from build123d import *

# Parameters (mm, degrees)
SKETCH1_W           = 50
SKETCH1_H           = 50
BOSS_EXTRUDE1_DEPTH = 30
BOSS_EXTRUDE2_DEPTH = 20
BOSS_EXTRUDE3_DEPTH = 20
CUT_EXTRUDE5_DEPTH  = 20
CUT_EXTRUDE6_DEPTH  = 20
CHAMFER1_SIZE       = 2
SKETCH4_R           = 3.1
CUT_EXTRUDE4_DEPTH  = 4
CHAMFER2_SIZE       = 1
CHAMFER3_SIZE       = 0.75
CHAMFER4_SIZE       = 2.5


with BuildPart() as part:
    # Sketch1 → Boss-Extrude1 (new body)
    with BuildSketch(Plane(origin=(0, 0, 0), x_dir=(1, 0, 0), z_dir=(0, 1, 0))):
        with Locations((25, 25)):
            Rectangle(SKETCH1_W, SKETCH1_H)
    extrude(amount=BOSS_EXTRUDE1_DEPTH)

    # Sketch3 → Boss-Extrude2 (add)
    with BuildSketch(Plane(origin=(0, 0, 0), x_dir=(1, 0, 0), z_dir=(0, 1, 0))):
        Polygon((50, 16.674315781), (50, 33.325684219), (52.3, 34.653589838), (52.3, 15.346410162), align=None)
    extrude(amount=BOSS_EXTRUDE2_DEPTH)

    # Sketch3_3 → Boss-Extrude3 (add)
    with BuildSketch(Plane(origin=(0, 0, 0), x_dir=(1, 0, 0), z_dir=(0, 1, 0))):
        Polygon((33.325684219, 50), (16.674315781, 50), (15.346410162, 52.3), (34.653589838, 52.3), align=None)
    extrude(amount=BOSS_EXTRUDE3_DEPTH)

    # Sketch3_6 → Cut-Extrude5 (cut)
    with BuildSketch(Plane(origin=(0, 0, 0), x_dir=(1, 0, 0), z_dir=(0, 1, 0))):
        Polygon((0, 33.787564435), (2.7, 35.346410162), (2.7, 14.653589838), (0, 16.212435565), align=None)
    extrude(amount=CUT_EXTRUDE5_DEPTH, mode=Mode.SUBTRACT)

    # Sketch3_7 → Cut-Extrude6 (cut)
    with BuildSketch(Plane(origin=(0, 0, 0), x_dir=(1, 0, 0), z_dir=(0, 1, 0))):
        Polygon((16.212435565, 0), (14.653589838, 2.7), (35.346410162, 2.7), (33.787564435, 0), align=None)
    extrude(amount=CUT_EXTRUDE6_DEPTH, mode=Mode.SUBTRACT)

    # Chamfer1
    chamfer1_edges = [part.edges().sort_by_distance(p)[0] for p in [
        (50, 30, -25),
        (25, 30, -50),
        (0, 30, -25),
        (25, 30, 0),
    ]]
    chamfer(chamfer1_edges, length=CHAMFER1_SIZE)

    # Sketch4 → Cut-Extrude4 (cut)
    with BuildSketch(Plane(origin=(0, 0, 0), x_dir=(1, 0, 0), z_dir=(0, 1, 0))):
        with Locations(Location((12.5, 37.5, 0), (0, 0, 270))):
            Circle(SKETCH4_R)
        with Locations(Location((37.5, 37.5, 0), (0, 0, 270))):
            Circle(SKETCH4_R)
        with Locations(Location((37.5, 12.5, 0), (0, 0, 270))):
            Circle(SKETCH4_R)
        with Locations(Location((12.5, 12.5, 0), (0, 0, 270))):
            Circle(SKETCH4_R)
    extrude(amount=CUT_EXTRUDE4_DEPTH, mode=Mode.SUBTRACT)

    # Chamfer2
    chamfer2_edges = [part.edges().sort_by_distance(p)[0] for p in [
        (12.5, 4, -15.6),
        (37.5, 4, -15.6),
        (37.5, 4, -40.6),
        (12.5, 4, -40.6),
    ]]
    chamfer(chamfer2_edges, length=CHAMFER2_SIZE)

    # Chamfer3
    chamfer3_edges = [part.edges().sort_by_distance(p)[0] for p in [
        (50, 0, -41.66284211),
        (51.15, 0, -16.010362971),
        (51.15, 0, -33.989637029),
        (52.3, 0, -25),
        (8.33715789, 0, -50),
        (33.989637029, 0, -51.15),
        (16.010362971, 0, -51.15),
        (25, 0, -52.3),
        (0, 0, -8.106217783),
        (1.35, 0, -15.433012702),
        (1.35, 0, -34.566987298),
        (2.7, 0, -25),
        (41.66284211, 0, -50),
        (41.893782217, 0, 0),
        (50, 0, -8.33715789),
        (34.566987298, 0, -1.35),
        (15.433012702, 0, -1.35),
        (8.106217783, 0, 0),
        (25, 0, -2.7),
        (0, 0, -41.893782217),
        (12.5, 0, -15.6),
        (37.5, 0, -15.6),
        (37.5, 0, -40.6),
        (12.5, 0, -40.6),
    ]]
    chamfer(chamfer3_edges, length=CHAMFER3_SIZE)

    # Chamfer4
    chamfer4_edges = [part.edges().sort_by_distance(p)[0] for p in [
        (0, 20, -25),
        (25, 20, 0),
    ]]
    chamfer(chamfer4_edges, length=CHAMFER4_SIZE)


solid = part.part
Model file for the job. Use its own axes, mm. A direction names the side the tool comes from. Coordinates: 2 decimals unless noted, no trailing zeros. Order: outer loops, then holes, each group sorted by start corner. A loop starts at its lowest first (then second) coordinate and runs counter-clockwise, first axis right, second up. Notation, with made-up numbers: (73, 11.5) -> (100, 11.5) arc R25 ccw to (100, 44.5) -> close; hole circle Ø2 at (12, 86.25). An arc over 180 degrees is marked (long way). Return JSON: item names as keys, results as strings. Group by question number.
Item 1: Saw through at D-D on x = 6.5. Write the cut outline in (y, z), then the cut area to 3 significant figures.
Item 2: Saw through at C-C on y = 7. Write the cut outline in (x, z).
Item 3: Saw through at B-B on x = 24. Write the cut outline in (y, z), then the cut area to 3 significant figures.
Item 4: Pull direction Z, two halves, no side cores. Call faces 1 (the flat face through (50.75, 0.38, -33.33)), 2 (the flat face through (1.331, 11.473, -34.556)), 3 (the flat face through (25, 20, -51)): pulls with the +Z half, pulls with the -Z half, needs draft (parallel to the pull), parting line crosses it, or undercut.
Item 5: Wall check: line 1 along X through (y, z) = (1.9, -12.5); line 2 along Z through (x, y) = (16, 5.5); line 3 along X through (y, z) = (13, -38.5). Give the ranges that are in metal, low to high. Write a range as [from, to].
Item 6: Tool access for faces 4 (the cylindrical face through (13.431, 1.859, -34.543)), 5 (the flat face through (25, 29, -1)): list every direction of +Z, -Z, +X, -X, +Y, -Y with a clear straight run to the whole face (end or side of a thin tool).
Item 7: Flat gauge pins, fed straight in: P1, Ø5, axis at x = 37.5, z = -37.5, coming from the -Y side; P2, Ø1.3, axis at x = 11.5, z = -38.5, coming from the -Y side; P3, Ø2.5, axis at x = 50.5, z = -27, coming from the +Y side. Where does each tip first touch, or does it go through?
Item 8: Saw through at A-A on z = -37.5. Write the cut outline in (x, y).
Values found:
{
 "1": {"outline": "(0, -49.25) -> (0.75, -50) -> (28, -50) -> (30, -48) -> (30, -2) -> (28, 0) -> (0.75, 0) -> (0, -0.75) -> close", "area": "1,500 mm2"},
 "2": {"outline": "(0, -50) -> (16.67, -50) -> (15.35, -52.3) -> (34.65, -52.3) -> (33.33, -50) -> (50, -50) -> (50, -33.33) -> (52.3, -34.65) -> (52.3, -15.35) -> (50, -16.67) -> (50, 0) -> (33.79, 0) -> (35.35, -2.7) -> (14.65, -2.7) -> (16.21, 0) -> (0, 0) -> (0, -16.21) -> (2.7, -14.65) -> (2.7, -35.35) -> (0, -33.79) -> close"},
 "3": {"outline": "(0, -51.55) -> (0.75, -52.3) -> (20, -52.3) -> (20, -50) -> (28, -50) -> (30, -48) -> (30, -2) -> (28, 0) -> (22.5, 0) -> (20, -2.5) -> (20, -2.7) -> (0.75, -2.7) -> (0, -3.45) -> close", "area": "1,480 mm2"},
 "4": {"face 1": "pulls with the -Z half", "face 2": "undercut", "face 3": "needs draft"},
 "5": {"line 1": "x = [0, 9.4], [15.6, 34.4], [40.6, 50]", "line 2": "z = [-52.3, -51.17], [-50, -2.7], [-0.37, 0]", "line 3": "x = [0, 50]"},
 "6": {"face 4": "-Y", "face 5": "+Z, +X, -X, +Y"},
 "7": {"P1": "stops at y = 3.6", "P2": "stops at y = 4", "P3": "stops at y = 28.75"},
 "8": {"outline": "(0, 0.75) -> (0.75, 0) -> (8.65, 0) -> (9.4, 0.75) -> (9.4, 3) -> (10.4, 4) -> (14.6, 4) -> (15.6, 3) -> (15.6, 0.75) -> (16.35, 0) -> (33.65, 0) -> (34.4, 0.75) -> (34.4, 3) -> (35.4, 4) -> (39.6, 4) -> (40.6, 3) -> (40.6, 0.75) -> (41.35, 0) -> (49.25, 0) -> (50, 0.75) -> (50, 28) -> (48, 30) -> (2, 30) -> (0, 28) -> close"}
}
